```python
from build123d import *

# Parameters (mm, degrees)
F0_R           = 6.875
F1_DEPTH       = 100
F3_D           = 2
F3_CBORE_D     = 6.25
F3_CBORE_DEPTH = 6.5
F4_R           = 1


with BuildPart() as f1:
    # F0 (on Top) → F1 (new body)
    with BuildSketch(Plane.XY):
        Circle(F0_R)
    extrude(amount=F1_DEPTH)

    # F3 (through all)
    with Locations(Plane(origin=(0, 0, 0), x_dir=(1, 0, 0), z_dir=(0, 0, -1))):
        with Locations((0, 0)):
            CounterBoreHole(F3_D / 2, F3_CBORE_D / 2, F3_CBORE_DEPTH)

    # F4
    f4_edges = [f1.edges().sort_by_distance(p)[0] for p in [
        (-6.875, 0, 100),
    ]]
    fillet(f4_edges, radius=F4_R)


solid = f1.part
```
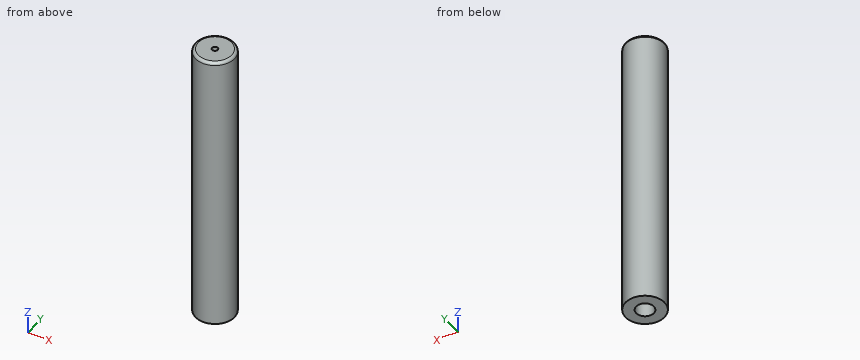
Build history of the part. All positions in model axes, mm. Give positions to 0.01 mm unless a question says otherwise; leave off trailing zeros. Loops run counter-clockwise (first coordinate to the right, second up) from the corner with the lowest first, then second, coordinate; pieces in that order, holes last. Notation, with made-up numbers: (43, 71) -> (51, 71) arc R18 ccw to (51, 76) -> close; hole circle Ø9 at (-1, -23). An arc over 180 degrees is marked (long way). One line per question, with ' | ' between items. Start each with the question number.
1) Cut at A-A (y = 0). Give the cut face in (x, z) (3 decimals), plus the area to 3 significant figures.
2) Probe L1, parallel to Y at x = 0, z = 74.5 (3 decimals); L2, parallel to Z at x = 1, y = -0.25; L3, parallel to Y at x = 3.5, z = 92.5. List the from-to ranges inside material, lowest first.
3) Pin check, flat tips, straight feed: pin 1 (8 mm diameter, centred on x = 3, z = 85, fed in from +Y) (3 decimals); pin 2 (1.5 mm diameter, centred on x = 1.5, z = 65, fed in from -Y); pin 3 (5.5 mm diameter, centred on x = 0, y = 0, fed in from -Z); pin 4 (5 mm diameter, centred on x = -5.5, z = 87.5, fed in from -Y). Stop position of each tip, or through.
4) Cut at C-C (z = 79). Give the cut face in (x, y) (3 decimals).
Return value:
1) outline: (-6.875, 0) -> (-3.125, 0) -> (-3.125, 6.5) -> (-1, 6.5) -> (-1, 100) -> (-5.875, 100) arc R1 ccw to (-6.875, 99) -> close; (1, 6.5) -> (3.125, 6.5) -> (3.125, 0) -> (6.875, 0) -> (6.875, 99) arc R1 ccw to (5.875, 100) -> (1, 100) -> close | area: 1,150 mm^2
2) L1: -6.875 to -1, 1 to 6.875 | L2: 6.5 to 100 | L3: -5.92 to 5.92
3) pin 1: y = 6.875 | pin 2: y = -6.83 | pin 3: z = 6.5 | pin 4: y = -6.19
4) outline: circle Ø13.75 at (0, 0); hole circle Ø2 at (0, 0)
